Work out the finished part from the listing and answer in its coordinate system (mm). A direction names the side the tool comes from. Give positions to 0.01 mm unless a question says otherwise; leave off trailing zeros. Write each loop counter-clockwise with the first axis right and the second up, starting at its lowest first coordinate (ties: lowest second). Pieces come first, ordered by that corner, then holes. Notation, with made-up numbers: (14, 52.25) -> (23, 52.25) arc R32 cw to (23, 89.25) -> close; hole circle Ø8 at (23, 18.5). An arc over 180 degrees is marked (long way). Use a Markdown table: item, result. Add a question column.
Q1. For faces 1 (the face through (0, 0, -180)), 2 (the face through (-3, 0, -7)), 3 (the face through (-3, 0, -103)), determine the directions among +Z, -Z, +X, -X, +Y, -Y from which every point of the face is accessible in a straight line to the end or side of a thin tool.
Q2. Section A-A, the plane z = -157.5 is taken. Give the vertices of the cut face in (x, y).
Q3. Each of these flat-tipped pins is pushed along its axis until it touches: pin 1 Ø2 at (x, z) = (1, -125) entering from +Y; pin 2 Ø2 at (y, z) = (2, -43) entering from -X; pin 3 Ø1 at (y, z) = (3, -143.5) entering from +X. Where does it stop, or does it pass through?
Q4. Consider line 1 (Y direction, x = -2.25, z = -37.5); line 2 (Z direction, x = 3.5, y = 0); line 3 (X direction, y = 2, z = -83.5). Determine where each line is inside the solid, lowest interval first.
Autodesk Inventor part; units mm, degrees
ref_plane "YZ Plane" through (0, 0, 0) normal (1, 0, 0) x (0, 1, 0)
ref_plane "XZ Plane" through (0, 0, 0) normal (0, 1, 0) x (-1, 0, 0)
ref_plane "XY Plane" through (0, 0, 0) normal (0, 0, 1) x (1, 0, 0)
sketch "Sketch1" plane through (0, 0, 0) normal (0, 1, 0) x (-1, 0, 0)
  line L0 (-3, -22) -> (-3, -180)
  line L1 (-3, -180) -> (0, -180)
  line L2 (0, -180) -> (0, 0)
  line L3 (-5, -18.5) -> (0, -18.5) construction
  line L4 (-5, -18.5) -> (-5, -20.565) construction
  line L5 (-3, -22) -> (-5, -18.5)
  line L6 (-5, -18.5) -> (-3, -15)
  line L7 (-3, -15) -> (-3, 0)
  line L8 (-3, 0) -> (0, 0)
  dimension "d5" = 180
  dimension "d8" = 5
  dimension "d12" = 6
  dimension "d14" = 15
  dimension "d15" = 7
revolve "Revolution1" add sketch "Sketch1" angle 360 about axis through (0, 0, -180) along (0, 0, 1)
fillet "Fillet2" radius 5 2 edges at (-3, 0, -22) (-3, 0, -15)
properties part number "SealantApplicator"
Result set:
| question | item | result |
|---|---|---|
| 1 | face 1 | -Z, +X, -X, +Y, -Y |
| 1 | face 2 | +Z |
| 1 | face 3 | -Z |
| 2 | outline | circle Ø6 at (0, 0) |
| 3 | pin 1 | stops at y = 3 |
| 3 | pin 2 | stops at x = -2.83 |
| 3 | pin 3 | stops at x = 1.66 |
| 4 | line 1 | y = -1.98 to 1.98 |
| 4 | line 2 | z = -21.15 to -15.85 |
| 4 | line 3 | x = -2.24 to 2.24 |
